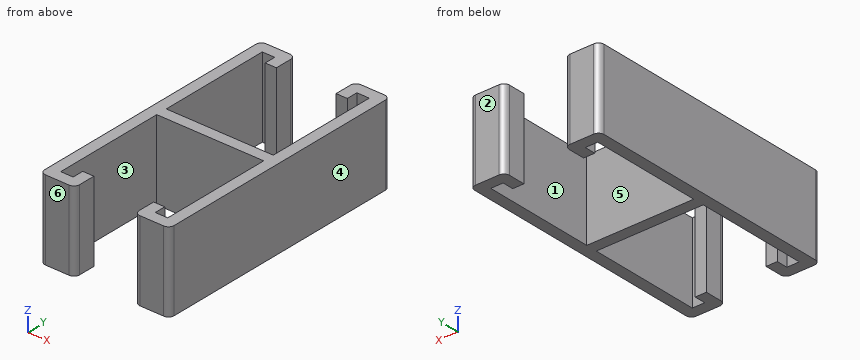
from build123d import *

# Parameters (mm, degrees)
BASE_EXTRUDE_DEPTH = 12.7


with BuildPart() as part:
    # Sketch1 → Base-Extrude (new, symmetric)
    with BuildSketch(Plane.XY):
        with BuildLine():
            Line((-11.3109375, 41.275), (-18.8515625, 41.275))
            ThreePointArc((-18.8515625, 41.275), (-20.114411017, 40.751911017), (-20.6375, 39.4890625))
            Line((-20.6375, 39.4890625), (-20.6375, -39.4890625))
            ThreePointArc((-20.6375, -39.4890625), (-20.114411017, -40.751911017), (-18.8515625, -41.275))
            Line((-18.8515625, -41.275), (-11.3109375, -41.275))
            ThreePointArc((-11.3109375, -41.275), (-10.048088983, -40.751911017), (-9.525, -39.4890625))
            Line((-9.525, -39.4890625), (-9.525, -34.13125))
            Line((-9.525, -34.13125), (-13.096875, -34.13125))
            Line((-13.096875, -34.13125), (-13.096875, -37.703125))
            Line((-13.096875, -37.703125), (-17.065625, -37.703125))
            Line((-17.065625, -37.703125), (-17.065625, -1.7859375))
            Line((-17.065625, -1.7859375), (17.065625, -1.7859375))
            Line((17.065625, -1.7859375), (17.065625, -37.703125))
            Line((17.065625, -37.703125), (13.096875, -37.703125))
            Line((13.096875, -37.703125), (13.096875, -34.13125))
            Line((13.096875, -34.13125), (9.525, -34.13125))
            Line((9.525, -34.13125), (9.525, -39.4890625))
            ThreePointArc((9.525, -39.4890625), (10.048088983, -40.751911017), (11.3109375, -41.275))
            Line((11.3109375, -41.275), (18.8515625, -41.275))
            ThreePointArc((18.8515625, -41.275), (20.114411017, -40.751911017), (20.6375, -39.4890625))
            Line((20.6375, -39.4890625), (20.6375, 39.4890625))
            ThreePointArc((20.6375, 39.4890625), (20.114411017, 40.751911017), (18.8515625, 41.275))
            Line((18.8515625, 41.275), (11.3109375, 41.275))
            ThreePointArc((11.3109375, 41.275), (10.048088983, 40.751911017), (9.525, 39.4890625))
            Line((9.525, 39.4890625), (9.525, 34.13125))
            Line((9.525, 34.13125), (13.096875, 34.13125))
            Line((13.096875, 34.13125), (13.096875, 37.703125))
            Line((13.096875, 37.703125), (17.065625, 37.703125))
            Line((17.065625, 37.703125), (17.065625, 1.7859375))
            Line((17.065625, 1.7859375), (-17.065625, 1.7859375))
            Line((-17.065625, 1.7859375), (-17.065625, 37.703125))
            Line((-17.065625, 37.703125), (-13.096875, 37.703125))
            Line((-13.096875, 37.703125), (-13.096875, 34.13125))
            Line((-13.096875, 34.13125), (-9.525, 34.13125))
            Line((-9.525, 34.13125), (-9.525, 39.4890625))
            ThreePointArc((-9.525, 39.4890625), (-10.048088983, 40.751911017), (-11.3109375, 41.275))
        make_face()
    extrude(amount=BASE_EXTRUDE_DEPTH, both=True)


solid = part.part
CAD build for the part. Positions are in the model's coordinates, mm. Face numbers are marked on the shaded views. A direction names the side the tool comes from. Round coordinates to 2 decimals unless told otherwise and drop trailing zeros. Write each loop counter-clockwise with the first axis right and the second up, starting at its lowest first coordinate (ties: lowest second). Pieces come first, ordered by that corner, then holes.
(1) Slice it at D-D, the plane x = -10.5. Write the cut outline in (y, z), and give its area (3 significant figures).
(2) Drop flat-ended pins along their axis: P1, Ø1, axis at x = -5.5, z = -9, coming from the +Y side; P2, Ø5, axis at x = 4.5, z = 0.5, coming from the -Y side; P3, Ø3, axis at x = 8.5, z = -5.5, coming from the +Y side. Give the stop position or say it passes through.
(3) Probe line 1 along Y through (x, z) = (-14, -6) (3 decimals); line 2 along Y through (x, z) = (13, 7.5) (3 decimals); line 3 along X through (y, z) = (-36, -6) (1 decimal). List the from-to ranges inside material, lowest first.
(4) Slice it at C-C, the plane x = 4.5. Write the cut outline in (y, z), and give its area (3 significant figures).
(5) Mould opens along X. For the marked faces 3, 4, 5 and 6 say: pulls with the +X half, pulls with the -X half, needs draft (parallel to the pull), parting line crosses it, or undercut.
(6) 3-axis set-ups, long thin cutter, end or side, ignore diameter. For the marked faces 1 and 2: which of +Z, -Z, +X, -X, +Y, -Y reach the whole face in a straight line?
(7) Slice it at A-A, the plane y = 15.5. Write the cut outline in (x, z).
(8) Slice it at B-B, the plane x = -15. Write the cut outline in (y, z) (3 decimals), and give its area (3 significant figures).
From the geometry:
1. outline: (-41.08, -12.7) - (-34.13, -12.7) - (-34.13, 12.7) - (-41.08, 12.7) - close; (-1.79, -12.7) - (1.79, -12.7) - (1.79, 12.7) - (-1.79, 12.7) - close; (34.13, -12.7) - (41.08, -12.7) - (41.08, 12.7) - (34.13, 12.7) - close
1. area: 444 mm2
2. P1: stops at y = 1.79
2. P2: stops at y = -1.79
2. P3: stops at y = 40.7
3. line 1: y = -41.275 to -37.703, -1.786 to 1.786, 37.703 to 41.275
3. line 2: y = -41.275 to -34.131, -1.786 to 1.786, 34.131 to 41.275
3. line 3: x = -20.6 to -17.1, -13.1 to -9.5, 9.5 to 13.1, 17.1 to 20.6
4. outline: (-1.79, -12.7) - (1.79, -12.7) - (1.79, 12.7) - (-1.79, 12.7) - close
4. area: 90.7 mm2
5. face 3: undercut
5. face 4: pulls with the +X half
5. face 5: undercut
5. face 6: needs draft
6. face 1: +Z, -Z
6. face 2: +Z, -Z, +X, -X, +Y
7. outline: (-20.64, -12.7) - (-17.07, -12.7) - (-17.07, 12.7) - (-20.64, 12.7) - close; (17.07, -12.7) - (20.64, -12.7) - (20.64, 12.7) - (17.07, 12.7) - close
8. outline: (-41.275, -12.7) - (-37.703, -12.7) - (-37.703, 12.7) - (-41.275, 12.7) - close; (-1.786, -12.7) - (1.786, -12.7) - (1.786, 12.7) - (-1.786, 12.7) - close; (37.703, -12.7) - (41.275, -12.7) - (41.275, 12.7) - (37.703, 12.7) - close
8. area: 272 mm2
